from build123d import *

# Parameters (mm, degrees)
F1_DEPTH = 25.4
F2_W     = 28.7031400949
F2_H     = 44.6516051888
F3_DEPTH = 25.4
F4_DEPTH = 25.4
F5_R     = 5.9098450102
F6_DEPTH = 106.9210470388
F7_W     = 27.7463691309
F7_H     = 9.0954080224
F7_H_2   = 14.3515700474
F8_DEPTH = 38.6391121352


with BuildPart() as f1:
    # F0 (on Top) → F1 (new body)
    with BuildSketch(Plane.XY):
        with BuildLine():
            Line((24.2865420878, -57.233504951), (24.2865420878, 57.233504951))
            Line((24.2865420878, 57.233504951), (11.6877524542, 57.233504951))
            ThreePointArc((11.6877524542, 57.233504951), (11.7283742061, 56.6995761613), (11.7419263642, 56.1642758548))
            ThreePointArc((11.7419263642, 56.1642758548), (0.6278652442, 45.5990671994), (-9.3614213529, 57.233504951))
            Line((-9.3614213529, 57.233504951), (-24.2865420878, 57.233504951))
            Line((-24.2865420878, 57.233504951), (-24.2865420878, -57.233504951))
            Line((-24.2865420878, -57.233504951), (-10.5787608136, -57.233504951))
            ThreePointArc((-10.5787608136, -57.233504951), (0, -46.6547441374), (10.5787608136, -57.233504951))
            Line((10.5787608136, -57.233504951), (24.2865420878, -57.233504951))
        make_face()
        with BuildLine():
            ThreePointArc((-24.2865420878, -57.233504951), (0, -81.5200470388), (24.2865420878, -57.233504951))
            Line((24.2865420878, -57.233504951), (10.5787608136, -57.233504951))
            ThreePointArc((10.5787608136, -57.233504951), (0, -67.8122657646), (-10.5787608136, -57.233504951))
            Line((-10.5787608136, -57.233504951), (-24.2865420878, -57.233504951))
        make_face()
        with BuildLine():
            Line((11.6877524542, 57.233504951), (24.2865420878, 57.233504951))
            ThreePointArc((24.2865420878, 57.233504951), (0, 81.5200470388), (-24.2865420878, 57.233504951))
            Line((-24.2865420878, 57.233504951), (-9.3614213529, 57.233504951))
            ThreePointArc((-9.3614213529, 57.233504951), (1.1631655507, 66.7430366684), (11.6877524542, 57.233504951))
        make_face()
    extrude(amount=F1_DEPTH)

    # F2 (on Front) → F3 (join)
    with BuildSketch(Plane.XZ):
        with Locations((0, 25.8776322007)):
            Rectangle(F2_W, F2_H)
        with BuildLine():
            Line((-14.3515700474, 48.2034347951), (14.3515700474, 48.2034347951))
            ThreePointArc((14.3515700474, 48.2034347951), (0, 62.5550048426), (-14.3515700474, 48.2034347951))
        make_face()
    extrude(amount=F3_DEPTH)

    # F4 (add): a face of the model
    f4_faces = [f1.faces().sort_by_distance(p)[0] for p in [
        (0, 0, 42.5881236801),
    ]]
    extrude(f4_faces, amount=F4_DEPTH)

    # F5 (on face) → F6 (cut, through all)
    with BuildSketch(Plane.XZ.offset(25.4)):
        with Locations((0, 48.2034347951)):
            Circle(F5_R)
    extrude(amount=-F6_DEPTH, mode=Mode.SUBTRACT)

    # F7 (on face) → F8 (cut, through all)
    with BuildSketch(Plane.YZ.offset(14.3515700474)):
        with BuildLine():
            Line((13.8731850311, 39.1080267727), (-13.8731840998, 39.1080267727))
            ThreePointArc((-13.8731840998, 39.1080267727), (4.657e-07, 30.2578937262), (13.8731850311, 39.1080267727))
        make_face()
        with Locations((4.657e-07, 43.6557307839)):
            Rectangle(F7_W, F7_H)
        with Locations((4.657e-07, 55.3792198189)):
            Rectangle(F7_W, F7_H_2)
    extrude(amount=-F8_DEPTH, mode=Mode.SUBTRACT)


solid = f1.part
Work out the finished part from the listing and answer in its coordinate system (mm). A direction names the side the tool comes from. Coordinates: 2 decimals unless noted, no trailing zeros. Write each loop counter-clockwise with the first axis right and the second up, starting at its lowest first coordinate (ties: lowest second). Pieces come first, ordered by that corner, then holes. Notation, with made-up numbers: M 25,62 L 70,62 A12 ccw 70,68 Z; hole C -38.5,-10.75 d5. An arc over 180 degrees is marked long. Answer as CSV lines item,"result". Start each with the question number.
Item 1: Consider L1, parallel to Z at x = 0, y = -21 (3 decimals); L2, parallel to Y at x = -14, z = 40; L3, parallel to Y at x = 0, z = 20. Determine where each line is inside the solid, lowest interval first.
Item 2: Flat-ended cylindrical pins translate along their axes: P1, Ø19, axis at x = 0, z = 48.2, coming from the +Y side; P2, Ø1, axis at x = 10.5, y = -36.5, coming from the -Z side; P3, Ø7, axis at x = 3, z = 54.5, coming from the -Y side; P4, Ø1.5, axis at y = -20, z = 53, coming from the +X side. Find the tip coordinate at first contact, or state that the pin passes through.
Item 3: Section A-A on z = 22.5 is taken. Write down the section's boundary in (x, y), and give its area (3 significant figures).
Item 4: A tool of negligible diameter and unlimited length cuts with its end or side. For faces 1 (the face through (14.352, 0, 29)), 2 (the face through (0, 25.4, 40)), 3 (the face through (-3, -13.873, 54)), 4 (the face through (-0.534, -81.514, 12.522)), 5 (the face through (-14.352, 0, 29)), from which of +Z, -Z, +X, -X, +Y, -Y can it reach the whole face along a straight path? Write none if from no direction.
Item 5: Determine the mould class of faces 6 (the face through (-2.293, -46.906, 12.522)), 7 (the face through (0, -25.4, 40)), 8 (the face through (3.4, 13.873, 53.3)), 9 (the face through (24.287, -1, 13)) for opening direction Y: released by +Y, released by -Y, zero draft, split by the parting line, or undercut.
Item 6: Section B-B on y = 65 is taken. Write down the section's boundary in (x, z), and give its area (3 significant figures).
Item 7: Section D-D on z = 56.5 is taken. Write down the section's boundary in (x, y).
Item 8: Section C-C on x = -4 is taken. Write down the section's boundary in (y, z), and give its area (3 significant figures).
Checks:
1,L1,"z = 0 to 42.294, 54.113 to 62.555"
1,L2,"y = -25.4 to -13.87, 13.87 to 25.4"
1,L3,"y = -81.52 to -67.81, -46.65 to 45.65, 66.68 to 81.52"
2,P1,"stops at y = 25.4"
2,P2,"stops at z = 0"
2,P3,"stops at y = -25.4"
2,P4,"stops at x = 13.77"
3,outline,"M -24.29,-57.23 A24.29 ccw 24.29,-57.23 L 24.29,57.23 A24.29 ccw -24.29,57.23 Z; hole C 0,-57.23 d21.16; hole C 1.16,56.16 d21.16"
3,area,"6,710 mm²"
4,face 1,"+Z, +X, +Y, -Y"
4,face 2,"+Z, +X, -X, +Y"
4,face 3,"+Z, +X, -X"
4,face 4,"+Z, -Z, -Y"
4,face 5,"+Z, -X, +Y, -Y"
5,face 6,"undercut"
5,face 7,"released by -Y"
5,face 8,"undercut"
5,face 9,"zero draft"
6,outline,"M -23.01,0 L -4.65,0 L -4.65,25.4 L -23.01,25.4 Z; M 6.98,0 L 23.01,0 L 23.01,25.4 L 6.98,25.4 Z"
6,area,"873 mm²"
7,outline,"M -11.71,-25.4 L 11.71,-25.4 L 11.71,-13.87 L -11.71,-13.87 Z; M -11.71,13.87 L 11.71,13.87 L 11.71,25.4 L -11.71,25.4 Z"
8,outline,"M -81.19,0 L -67.03,0 L -67.03,25.4 L -81.19,25.4 Z; M -47.44,0 L 46.93,0 L 46.93,25.4 L 25.4,25.4 L 25.4,43.85 L 13.87,43.85 L 13.87,39.11 A15.3 cw -13.87,39.11 L -13.87,43.85 L -25.4,43.85 L -25.4,25.4 L -47.44,25.4 Z; M -25.4,52.55 L -13.87,52.55 L -13.87,61.99 L -25.4,61.99 Z; M 13.87,52.55 L 25.4,52.55 L 25.4,61.99 L 13.87,61.99 Z; M 65.4,0 L 81.19,0 L 81.19,25.4 L 65.4,25.4 Z"
8,area,"4,000 mm²"
